```python
from build123d import *

# Parameters (mm, degrees)
SKETCH2_R           = 3.048
BOSS_EXTRUDE1_DEPTH = 5.07492
CUT_EXTRUDE11_DEPTH = 210.646067011
SKETCH3_R           = 6.35
SKETCH3_R_2         = 2.032
CUT_EXTRUDE12_DEPTH = 210.646067011
SKETCH5_R           = 1.4732
CUT_EXTRUDE13_DEPTH = 210.646067011
SKETCH7_R           = 1.905
CUT_EXTRUDE14_DEPTH = 210.646067011
SKETCH8_R           = 3.175
CUT_EXTRUDE15_DEPTH = 210.646067011
SKETCH9_W           = 38.1
SKETCH9_H           = 63.5
CUT_EXTRUDE16_DEPTH = 5.08


with BuildPart() as part:
    # Sketch2 → Boss-Extrude1 (new body)
    with BuildSketch(Plane.XY):
        with BuildLine():
            Line((-186.69, -31.75), (-144.826640797, -31.75))
            ThreePointArc((-144.826640797, -31.75), (-123.19, -59.055), (-101.553359203, -31.75))
            Line((-101.553359203, -31.75), (101.553359203, -31.75))
            ThreePointArc((101.553359203, -31.75), (123.19, -59.055), (144.826640797, -31.75))
            Line((144.826640797, -31.75), (186.69, -31.75))
            Line((186.69, -31.75), (186.69, 95.25))
            Line((186.69, 95.25), (-186.69, 95.25))
            Line((-186.69, 95.25), (-186.69, -31.75))
        make_face()
        with Locations((-86.868, -16.51)):
            Circle(SKETCH2_R, mode=Mode.SUBTRACT)
        with Locations((86.868, -16.51)):
            Circle(SKETCH2_R, mode=Mode.SUBTRACT)
        with Locations((123.19, 76.2)):
            Circle(SKETCH2_R, mode=Mode.SUBTRACT)
        with Locations((-123.19, 76.2)):
            Circle(SKETCH2_R, mode=Mode.SUBTRACT)
    extrude(amount=-BOSS_EXTRUDE1_DEPTH)

    # Sketch2_4 → Cut-Extrude11 (cut, through all)
    with BuildSketch(Plane.XY):
        with BuildLine():
            ThreePointArc((-119.486801079, -31.75), (-123.19, -30.5435), (-126.893198921, -31.75))
            Line((-126.893198921, -31.75), (-119.486801079, -31.75))
        make_face()
        with BuildLine():
            Line((-119.486801079, -31.75), (-126.893198921, -31.75))
            ThreePointArc((-126.893198921, -31.75), (-126.039554547, -42.433581099), (-116.9035, -36.83))
            ThreePointArc((-116.9035, -36.83), (-117.586418901, -33.980445453), (-119.486801079, -31.75))
        make_face()
        with BuildLine():
            ThreePointArc((126.893198921, -31.75), (123.19, -30.5435), (119.486801079, -31.75))
            Line((119.486801079, -31.75), (126.893198921, -31.75))
        make_face()
        with BuildLine():
            Line((126.893198921, -31.75), (119.486801079, -31.75))
            ThreePointArc((119.486801079, -31.75), (120.340445453, -42.433581099), (129.4765, -36.83))
            ThreePointArc((129.4765, -36.83), (128.793581099, -33.980445453), (126.893198921, -31.75))
        make_face()
    extrude(amount=-CUT_EXTRUDE11_DEPTH, mode=Mode.SUBTRACT)

    # Sketch3 → Cut-Extrude12 (cut, through all)
    with BuildSketch(Plane.XY):
        with Locations((-10.209304394, 52.890523875)):
            Circle(SKETCH3_R)
        with Locations((7.316695606, 52.890523875)):
            Circle(SKETCH3_R_2)
        with Locations((52.574132234, 1.27)):
            Circle(SKETCH3_R)
        with Locations((70.100132234, 1.27)):
            Circle(SKETCH3_R_2)
        with Locations((52.574132234, 18.796)):
            Circle(SKETCH3_R_2)
        with Locations((35.048132234, 1.27)):
            Circle(SKETCH3_R_2)
        with Locations((-10.209304394, 70.416523875)):
            Circle(SKETCH3_R_2)
        with Locations((-27.735304394, 52.890523875)):
            Circle(SKETCH3_R_2)
        with Locations((-10.209304394, 35.364523875)):
            Circle(SKETCH3_R_2)
        with Locations((52.574132234, -16.256)):
            Circle(SKETCH3_R_2)
    extrude(amount=-CUT_EXTRUDE12_DEPTH, mode=Mode.SUBTRACT)

    # Sketch5 → Cut-Extrude13 (cut, through all)
    with BuildSketch(Plane.XY):
        with Locations((-30.346455717, 29.672559007)):
            Circle(SKETCH5_R)
        with Locations((9.927846929, 29.672559007)):
            Circle(SKETCH5_R)
        with Locations((-40.393083971, 47.101032839)):
            Circle(SKETCH5_R)
        with Locations((19.974475183, 47.101032839)):
            Circle(SKETCH5_R)
        with Locations((32.436980911, -21.947964868)):
            Circle(SKETCH5_R)
        with Locations((72.711283557, -21.947964868)):
            Circle(SKETCH5_R)
        with Locations((22.390352657, -4.519491037)):
            Circle(SKETCH5_R)
        with Locations((82.757911811, -4.519491037)):
            Circle(SKETCH5_R)
    extrude(amount=-CUT_EXTRUDE13_DEPTH, mode=Mode.SUBTRACT)

    # Sketch7 → Cut-Extrude14 (cut, through all)
    with BuildSketch(Plane.XY):
        with Locations((131.572, -19.05)):
            Circle(SKETCH7_R)
        with Locations((114.808, -19.05)):
            Circle(SKETCH7_R)
        with Locations((-123.19, -49.022)):
            Circle(SKETCH7_R)
        with Locations((-131.572, -19.05)):
            Circle(SKETCH7_R)
        with Locations((-114.808, -19.05)):
            Circle(SKETCH7_R)
        with Locations((123.19, -49.022)):
            Circle(SKETCH7_R)
    extrude(amount=-CUT_EXTRUDE14_DEPTH, mode=Mode.SUBTRACT)

    # Sketch8 → Cut-Extrude15 (cut, through all)
    with BuildSketch(Plane.XY):
        with Locations((0, -23.114)):
            Circle(SKETCH8_R)
    extrude(amount=-CUT_EXTRUDE15_DEPTH, mode=Mode.SUBTRACT)

    # Sketch9 → Cut-Extrude16 (cut)
    with BuildSketch(Plane.XY):
        with Locations((167.64, 63.5)):
            Rectangle(SKETCH9_W, SKETCH9_H)
    extrude(amount=-CUT_EXTRUDE16_DEPTH, mode=Mode.SUBTRACT)


solid = part.part
```
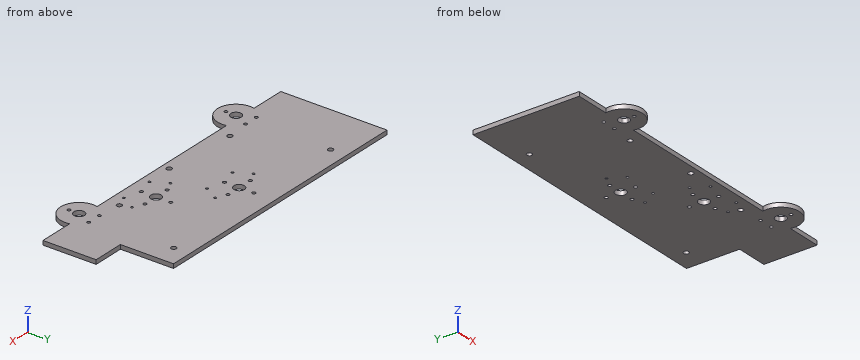
For this review, take the finished solid that the model builds, in its own axes (mm). Round coordinates to 2 decimals unless told otherwise and drop trailing zeros. Order: outer loops, then holes, each group sorted by start corner. A loop starts at its lowest first (then second) coordinate and runs counter-clockwise, first axis right, second up. Notation, with made-up numbers: (35.25, -21.5) -> (89.25, -21.5) arc R19 cw to (89.25, 10.5) -> close; hole circle Ø10 at (66.5, -33.5). An arc over 180 degrees is marked (long way). Use a Markdown table: item, result.
Item 1: Take a section at A-A (x = -35.5). State the section outline as (y, z) points, plus the area to 3 significant figures.
Resolved:
| item | result |
|---|---|
| outline | (-31.75, -5.07) -> (95.25, -5.07) -> (95.25, 0) -> (-31.75, 0) -> close |
| area | 645 mm² |
Item 2: For line 1 along X through (y, z) = (2.5, -0.4); line 2 along X through (y, z) = (75, -1.4); line 3 along X through (y, z) = (67, -2.25), list the stretches that pass through material, from the lowest coordinate up. Write a range as [from, to].
Resolved:
| item | result |
|---|---|
| line 1 | x = [-186.69, 33.43], [36.67, 46.34], [58.8, 68.48], [71.72, 186.69] |
| line 2 | x = [-186.69, -125.99], [-120.39, 120.39], [125.99, 148.59] |
| line 3 | x = [-186.69, 148.59] |
Item 3: Take a section at B-B (z = -2.75). State how many separate pieces and enclosed holes the cut face has, plus the area to 3 significant figures.
Resolved:
| item | result |
|---|---|
| separate pieces | 1 |
| enclosed holes | 31 |
| area | 46,100 mm² |
Item 4: For pin 1 (1 mm diameter, centred on x = 36.5, z = -2, fed in from -Y), flat-tipped, find the tip position at first contact; note if it passes through.
Resolved:
| item | result |
|---|---|
| pin 1 | stops at y = -31.75 |
